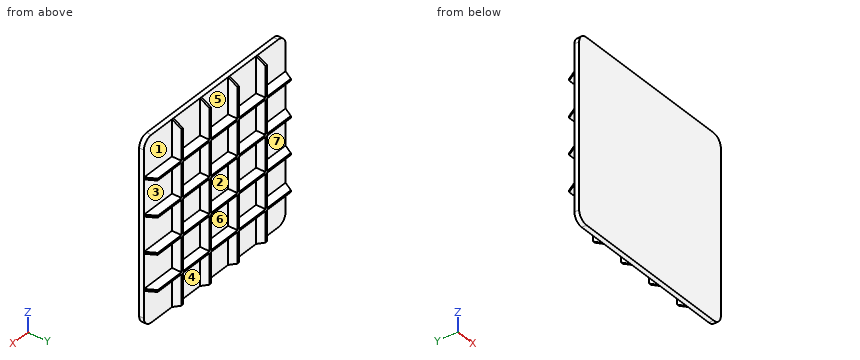
Autodesk Fusion 360 part; units mm, degrees
sketch "スケッチ1" plane through (0, 0, 0) normal (0, 1, 0) x (1, 0, 0)
  line L0 (1, 0) -> (18.2, 0)
  line L1 (19.2, -1) -> (19.2, -18.2)
  line L2 (18.2, -19.2) -> (1, -19.2)
  line L3 (0, -18.2) -> (0, -1)
  line L4 (3.8, -19.2) -> (3.8, 0)
  line L5 (4, -19.2) -> (4, 0)
  line L6 (7.6, 0) -> (7.6, -19.2)
  line L7 (7.8, -19.2) -> (7.8, 0)
  line L8 (19.2, -3.8) -> (0, -3.8)
  line L9 (0, -4) -> (19.2, -4)
  line L10 (19.2, -7.6) -> (0, -7.6)
  line L11 (0, -7.8) -> (19.2, -7.8)
  line L12 (0, -11.4) -> (19.2, -11.4)
  line L13 (19.2, -11.6) -> (0, -11.6)
  line L14 (0, -15.2) -> (19.2, -15.2)
  line L15 (19.2, -15.4) -> (0, -15.4)
  line L16 (11.4, -19.2) -> (11.4, 0)
  line L17 (11.6, 0) -> (11.6, -19.2)
  line L18 (15.2, -19.2) -> (15.2, 0)
  line L19 (15.4, 0) -> (15.4, -19.2)
  arc A0 (18.2, -19.2) -> (19.2, -18.2) centre (18.2, -18.2) ccw
  arc A1 (19.2, -1) -> (18.2, 0) centre (18.2, -1) ccw
  arc A2 (1, 0) -> (0, -1) centre (1, -1) ccw
  arc A3 (0, -18.2) -> (1, -19.2) centre (1, -18.2) ccw
  line L20 (-20.3302, 0) -> (25.6829, 0) construction
  line L21 (0, -22.3952) -> (0, 11.1848) construction
  dimension "d3" = 3.8
  dimension "d5" = 3.6
  dimension "d6" = 0.2
  dimension "d7" = 3.8
  dimension "d8" = 0.2
  dimension "d9" = 3.6
  dimension "d10" = 0.2
  dimension "d11" = 0.2
  dimension "d12" = 3.6
  dimension "d13" = 0.2
  dimension "d14" = 3.6
  dimension "d15" = 0.2
  dimension "d16" = 3.6
  dimension "d17" = 0.2
  dimension "d18" = 0.2
  dimension "d19" = 3.6
  dimension "d24" = 3.8
  dimension "d25" = 3.8
  dimension "d34" = 1
extrude "押し出し1" add sketch "スケッチ1" along normal blind 0.5 contours L0 L3 L4 L8 A2 | L0 L5 L6 L8 | L3 L4 L9 L10 | L0 L7 L8 L16 | L5 L6 L9 L10 | L3 L4 L11 L12 | L0 L8 L17 L18 | L7 L9 L10 L16 | L5 L6 L11 L12 | L3 L4 L13 L14 | L0 L1 L8 L19 A1 | L9 L10 L17 L18 | L7 L11 L12 L16 | L5 L6 L13 L14 | L2 L3 L4 L15 A3 | L1 L9 L10 L19 | L11 L12 L17 L18 | L7 L13 L14 L16 | L2 L5 L6 L15 | L1 L11 L12 L19 | L13 L14 L17 L18 | L2 L7 L15 L16 | L1 L13 L14 L19 | L2 L15 L17 L18 | L1 L2 L15 L19 A0 makes body 1 at (9, 0, 5.2) makes body 2 at (17.9333, 0, 2.8667) makes body 3 at (9, 0, 2.5333) makes body 4 at (10.2, 0, 14) makes body 5 at (5.2, 0, 5.2) makes body 6 at (1.2667, 0, 9) makes body 7 at (2.5333, 0, 14) makes body 8 at (6.4, 0, 1.2667) makes body 9 at (6.4, 0, 14) makes body 10 at (9, 0, 9) makes body 11 at (12.8, 0, 5.2) makes body 12 at (16.6667, 0, 9) makes body 13 at (14, 0, 14) makes body 14 at (12.8, 0, 9) makes body 15 at (12.8, 0, 2.5333) makes body 16 at (1.2667, 0, 5.2) makes body 17 at (5.2, 0, 9) makes body 18 at (16.6667, 0, 5.2) makes body 19 at (1.2667, 0, 16.3333) makes body 20 at (2.8667, 0, 1.2667) makes body 21 at (17.9333, 0, 14) makes body 22 at (17.9333, 0, 16.3333) makes body 23 at (9, 0, 17.9333) makes body 24 at (5.2, 0, 16.6667) makes body 25 at (12.8, 0, 17.9333)
extrude "押し出し2" add sketch "スケッチ1" along normal blind 1.5 contours L0 L4 L5 L8 | L4 L5 L8 L9 | L3 L4 L8 L9 | L0 L6 L7 L8 | L5 L6 L8 L9 | L4 L5 L9 L10 | L6 L7 L8 L9 | L4 L5 L10 L11 | L3 L4 L10 L11 | L0 L8 L16 L17 | L7 L8 L9 L16 | L6 L7 L9 L10 | L5 L6 L10 L11 | L4 L5 L11 L12 | L8 L9 L16 L17 | L6 L7 L10 L11 | L4 L5 L12 L13 | L3 L4 L12 L13 | L0 L8 L18 L19 | L8 L9 L17 L18 | L9 L10 L16 L17 | L7 L10 L11 L16 | L6 L7 L11 L12 | L5 L6 L12 L13 | L4 L5 L13 L14 | L8 L9 L18 L19 | L10 L11 L16 L17 | L6 L7 L12 L13 | L4 L5 L14 L15 | L3 L4 L14 L15 | L1 L8 L9 L19 | L9 L10 L18 L19 | L10 L11 L17 L18 | L11 L12 L16 L17 | L7 L12 L13 L16 | L6 L7 L13 L14 | L5 L6 L14 L15 | L2 L4 L5 L15 | L10 L11 L18 L19 | L12 L13 L16 L17 | L6 L7 L14 L15 | L1 L10 L11 L19 | L11 L12 L18 L19 | L12 L13 L17 L18 | L13 L14 L16 L17 | L7 L14 L15 L16 | L2 L6 L7 L15 | L12 L13 L18 L19 | L14 L15 L16 L17 | L1 L12 L13 L19 | L13 L14 L18 L19 | L14 L15 L17 L18 | L2 L15 L16 L17 | L14 L15 L18 L19 | L1 L14 L15 L19 | L2 L15 L18 L19 bodies 1 2 3 4 5 6 7 8 9 10 11 12 13 14 15 16 17 18 19 20 21 22 23 24 25
sketch "スケッチ5" plane through (15.4, 0, 0) normal (1, 0, 0) x (0, 0, -1)
  line L0 (-19.2, 0.5) -> (-15.4, 0.5)
  line L1 (-15.4, 0.5) -> (-15.4, 1.5)
  line L2 (-15.4, 1.5) -> (-19.2, 1.5)
  line L3 (-19.2, 1.5) -> (-19.2, 0.5)
  line L4 (-19.2, 0.5) -> (-16.9184, 4.4518)
  line L5 (-16.9184, 4.4518) -> (-19.2, 4.4518)
  line L6 (-19.2, 4.4518) -> (-19.2, 0.5)
  dimension "d35" = 30
sketch "スケッチ6" plane through (15.4, 0, 0) normal (1, 0, 0) x (0, 0, -1)
  line L0 (-3.8, 0.5) -> (0, 0.5)
  line L1 (0, 0.5) -> (0, 1.5)
  line L2 (0, 1.5) -> (-3.8, 1.5)
  line L3 (-3.8, 1.5) -> (-3.8, 0.5)
  line L4 (0, 0.5) -> (0, 4.8319)
  line L5 (0, 4.8319) -> (-2.501, 4.8319)
  line L6 (-2.501, 4.8319) -> (0, 0.5)
  dimension "d36" = 30
extrude "押し出し5" cut sketch "スケッチ6" sketch "スケッチ5" against normal blind 14.5 contours L1 L2 L4 L6 of sketch 2 contours L2 L3 L4 L6 bodies 1
sketch "スケッチ3" plane through (0, 0, 15.4) normal (0, 0, 1) x (1, 0, 0)
  line L0 (0, 0.5) -> (3.8, 0.5)
  line L1 (3.8, 0.5) -> (3.8, 1.5)
  line L2 (3.8, 1.5) -> (0, 1.5)
  line L3 (0, 1.5) -> (0, 0.5)
  line L4 (0, 0.5) -> (0, 2.6672)
  line L5 (0, 2.6672) -> (1.2513, 2.6672)
  line L6 (1.2513, 2.6672) -> (0, 0.5)
  dimension "d30" = 30
sketch "スケッチ4" plane through (0, 0, 15.4) normal (0, 0, 1) x (1, 0, 0)
  line L0 (15.4, 0.5) -> (19.2, 0.5)
  line L1 (19.2, 0.5) -> (19.2, 1.5)
  line L2 (19.2, 1.5) -> (15.4, 1.5)
  line L3 (15.4, 1.5) -> (15.4, 0.5)
  line L4 (19.2, 0.5) -> (19.2, 2.9821)
  line L5 (19.2, 2.9821) -> (17.7669, 2.9821)
  line L6 (17.7669, 2.9821) -> (19.2, 0.5)
  dimension "d31" = 30
extrude "押し出し4" cut sketch "スケッチ3" sketch "スケッチ4" against normal blind 13 contours L2 L3 L4 L6 | L2 L4 L5 L6 of sketch 2 contours L1 L2 L4 L6 | L2 L4 L5 L6 bodies 1
Build history of the part. All positions in model axes, mm. Face numbers are marked on the shaded views. A direction names the side the tool comes from. Coordinates: 2 decimals unless noted, no trailing zeros. Order: outer loops, then holes, each group sorted by start corner. A loop starts at its lowest first (then second) coordinate and runs counter-clockwise, first axis right, second up.
Item 1: Drill centre lines: L1, parallel to Z at x = 17.5, y = 1.25; L2, parallel to Y at x = 12.75, z = 16.5. Where is each one in solid material? Low to high.
Filled in:
L1: z = 3.8 to 4, 7.6 to 7.8, 11.4 to 11.6, 15.2 to 15.4
L2: y = 0 to 0.5
Item 2: Mould opens along Z. For the marked faces 1 and 2 say: released by +Z, released by -Z, zero draft, split by the parting line, or undercut.
Filled in:
face 1: zero draft
face 2: undercut
Item 3: Saw through at B-B on z = 3.25. List the corners of the cut face in (x, y).
Filled in:
outline: (0, 0) - (19.2, 0) - (19.2, 0.5) - (15.4, 0.5) - (15.4, 1.5) - (15.2, 1.5) - (15.2, 0.5) - (11.6, 0.5) - (11.6, 1.5) - (11.4, 1.5) - (11.4, 0.5) - (7.8, 0.5) - (7.8, 1.5) - (7.6, 1.5) - (7.6, 0.5) - (4, 0.5) - (4, 1.5) - (3.8, 1.5) - (3.8, 0.5) - (0, 0.5) - close
Item 4: Saw through at A-A on x = 9.5. List the corners of the cut face in (y, z), then the cut area to 3 significant figures.
Filled in:
outline: (0, 0) - (0.5, 0) - (0.5, 3.8) - (1.5, 3.8) - (1.5, 4) - (0.5, 4) - (0.5, 7.6) - (1.5, 7.6) - (1.5, 7.8) - (0.5, 7.8) - (0.5, 11.4) - (1.5, 11.4) - (1.5, 11.6) - (0.5, 11.6) - (0.5, 15.2) - (1.5, 15.2) - (1.5, 15.4) - (0.5, 15.4) - (0.5, 19.2) - (0, 19.2) - close
area: 10.4 mm2
Item 5: Drop flat-ended pins along their axis: pin 1 Ø0.8 at (x, y) = (6, 1) entering from +Z; pin 2 Ø1.1 at (x, z) = (14.5, 2.5) entering from +Y; pin 3 Ø0.5 at (y, z) = (1, 5.5) entering from +X. Give the stop position or say it passes through.
Filled in:
pin 1: stops at z = 15.4
pin 2: stops at y = 0.5
pin 3: stops at x = 15.4
Item 6: Tool access for the marked faces 3, 4, 5, 6 and 7: list every direction of +Z, -Z, +X, -X, +Y, -Y with a clear straight run to the whole face (end or side of a thin tool).
Filled in:
face 3: +X, +Y
face 4: -Z, +Y
face 5: +Z, +Y
face 6: +Y
face 7: -X, +Y
Item 7: Saw through at C-C on y = 1. State how many separate pieces and enclosed holes the cut face has, then the cut area to 3 significant figures.
Filled in:
separate pieces: 1
enclosed holes: 9
area: 29.2 mm2
